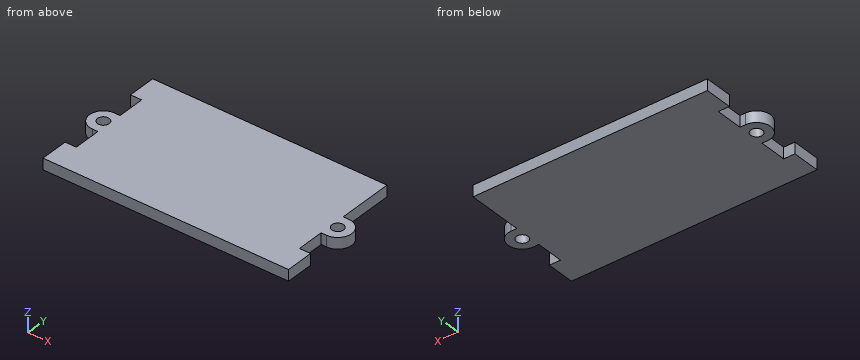
from build123d import *

# Parameters (mm, degrees)
ESQUISSE1_W             = 80
ESQUISSE1_H             = 49.614813968
BOSS_EXTRU_1_DEPTH      = 4
ESQUISSE3_W             = 4
ESQUISSE3_H             = 10
BOSS_EXTRU_3_DEPTH      = 4
ESQUISSE4_R             = 2.1
ENL_V_MAT_EXTRU_1_DEPTH = 101.232877665


with BuildPart() as part:
    # Esquisse1 → Boss.-Extru.1 (new body)
    with BuildSketch(Plane.XY):
        with Locations((40, 24.807406984)):
            Rectangle(ESQUISSE1_W, ESQUISSE1_H)
    extrude(amount=BOSS_EXTRU_1_DEPTH)

    # Esquisse3 → Boss.-Extru.3 (add)
    with BuildSketch(Plane(origin=(0, 0, 4), x_dir=(-1, 0, 0), z_dir=(0, 0, -1))):
        with Locations((2, 5)):
            Rectangle(ESQUISSE3_W, ESQUISSE3_H)
        with BuildLine():
            Line((0, 19.807406984), (2, 19.807406984))
            ThreePointArc((2, 19.807406984), (7, 24.807406984), (2, 29.807406984))
            Line((2, 29.807406984), (0, 29.807406984))
            Line((0, 29.807406984), (0, 19.807406984))
        make_face()
        with Locations((2, 44.614813968)):
            Rectangle(ESQUISSE3_W, ESQUISSE3_H)
        with BuildLine():
            Line((-80, 29.807406984), (-82, 29.807406984))
            ThreePointArc((-82, 29.807406984), (-87, 24.807406984), (-82, 19.807406984))
            Line((-82, 19.807406984), (-80, 19.807406984))
            Line((-80, 19.807406984), (-80, 29.807406984))
        make_face()
        with Locations((-82, 5)):
            Rectangle(ESQUISSE3_W, ESQUISSE3_H)
    extrude(amount=BOSS_EXTRU_3_DEPTH)

    # Esquisse4 → Enlèv. mat.-Extru.1 (cut, through all)
    with BuildSketch(Plane(origin=(0, 0, 0), x_dir=(-1, 0, 0), z_dir=(0, 0, -1))):
        with Locations((2, 24.807406984)):
            Circle(ESQUISSE4_R)
        with Locations((-82, 24.807406984)):
            Circle(ESQUISSE4_R)
    extrude(amount=-ENL_V_MAT_EXTRU_1_DEPTH, mode=Mode.SUBTRACT)


solid = part.part
Design review of the part built by this model. Coordinates are the model's own, in mm. Give positions to 0.01 mm unless a question says otherwise; leave off trailing zeros. Loops run counter-clockwise (first coordinate to the right, second up) from the corner with the lowest first, then second, coordinate; pieces in that order, holes last. Notation, with made-up numbers: M -12.75,79.5 L -3.75,79.5 A18 ccw -3.75,93.5 Z; hole C 76,9 d7. An arc over 180 degrees is marked long. Answer as a JSON object with one key per item and string values.
Item 1: We need section C-C (y = 44). State the section outline as (x, z) points, and give its area (3 significant figures).
Output values:
{"outline": "M -4,0 L 80,0 L 80,4 L -4,4 Z", "area": "336 mm2"}
Item 2: We need section A-A (z = 0.7). State the section outline as (x, y) points, and give its area (3 significant figures).
Output values:
{"outline": "M -4,0 L 84,0 L 84,10 L 80,10 L 80,19.81 L 82,19.81 A5 ccw 82,29.81 L 80,29.81 L 80,49.61 L -4,49.61 L -4,39.61 L 0,39.61 L 0,29.81 L -2,29.81 A5 ccw -2,19.81 L 0,19.81 L 0,10 L -4,10 Z; hole C -2,24.81 d4.2; hole C 82,24.81 d4.2", "area": "4,180 mm2"}
Item 3: We need section B-B (y = 38.5). State the section outline as (x, z) points, and give its area (3 significant figures).
Output values:
{"outline": "M 0,0 L 80,0 L 80,4 L 0,4 Z", "area": "320 mm2"}
Item 4: Wall thickness on line 1 along Y through (x, z) = (-2, 3.05); line 2 along Y through (x, z) = (82, 1.3); line 3 along X through (y, z) = (30, 3.1): over which ranges is each line inside the solid? List them lowest first.
Output values:
{"line 1": "y = 0 to 10, 19.81 to 22.71, 26.91 to 29.81, 39.61 to 49.61", "line 2": "y = 0 to 10, 19.81 to 22.71, 26.91 to 29.81", "line 3": "x = 0 to 80"}
Item 5: For P1, Ø2, axis at y = 3, z = 2.5, coming from the -X side; P2, Ø1, axis at x = 81, z = 2.5, coming from the +Y side; P3, Ø1.2, axis at y = 2.5, z = 1.5, coming from the +X side, all flat-tipped, find the tip position at first contact; note any pin that passes through.
Output values:
{"P1": "stops at x = -4", "P2": "stops at y = 29.81", "P3": "stops at x = 84"}
